from build123d import *

# Parameters (mm, degrees)
SKETCH1_R           = 1.5
BOSS_EXTRUDE1_DEPTH = 3


with BuildPart() as part:
    # Sketch1 → Boss-Extrude1 (new body)
    with BuildSketch(Plane.XY):
        with BuildLine():
            Line((-105, 15), (105, 15))
            ThreePointArc((105, 15), (112.071067812, 12.071067812), (115, 5))
            Line((115, 5), (115, -5))
            ThreePointArc((115, -5), (112.071067812, -12.071067812), (105, -15))
            Line((105, -15), (-105, -15))
            ThreePointArc((-105, -15), (-112.071067812, -12.071067812), (-115, -5))
            Line((-115, -5), (-115, 5))
            ThreePointArc((-115, 5), (-112.071067812, 12.071067812), (-105, 15))
        make_face()
        with Locations((-105, 5)):
            Circle(SKETCH1_R, mode=Mode.SUBTRACT)
        with Locations((-95, 5)):
            Circle(SKETCH1_R, mode=Mode.SUBTRACT)
        with Locations((-85, 5)):
            Circle(SKETCH1_R, mode=Mode.SUBTRACT)
        with Locations((-75, 5)):
            Circle(SKETCH1_R, mode=Mode.SUBTRACT)
        with Locations((-65, 5)):
            Circle(SKETCH1_R, mode=Mode.SUBTRACT)
        with Locations((-55, 5)):
            Circle(SKETCH1_R, mode=Mode.SUBTRACT)
        with Locations((-45, 5)):
            Circle(SKETCH1_R, mode=Mode.SUBTRACT)
        with Locations((-35, 5)):
            Circle(SKETCH1_R, mode=Mode.SUBTRACT)
        with Locations((-25, 5)):
            Circle(SKETCH1_R, mode=Mode.SUBTRACT)
        with Locations((-15, 5)):
            Circle(SKETCH1_R, mode=Mode.SUBTRACT)
        with Locations((-5, 5)):
            Circle(SKETCH1_R, mode=Mode.SUBTRACT)
        with Locations((15, 5)):
            Circle(SKETCH1_R, mode=Mode.SUBTRACT)
        with Locations((25, 5)):
            Circle(SKETCH1_R, mode=Mode.SUBTRACT)
        with Locations((5, 5)):
            Circle(SKETCH1_R, mode=Mode.SUBTRACT)
        with Locations((35, 5)):
            Circle(SKETCH1_R, mode=Mode.SUBTRACT)
        with Locations((45, 5)):
            Circle(SKETCH1_R, mode=Mode.SUBTRACT)
        with Locations((55, 5)):
            Circle(SKETCH1_R, mode=Mode.SUBTRACT)
        with Locations((65, 5)):
            Circle(SKETCH1_R, mode=Mode.SUBTRACT)
        with Locations((75, 5)):
            Circle(SKETCH1_R, mode=Mode.SUBTRACT)
        with Locations((85, 5)):
            Circle(SKETCH1_R, mode=Mode.SUBTRACT)
        with Locations((95, 5)):
            Circle(SKETCH1_R, mode=Mode.SUBTRACT)
        with Locations((-85, -5)):
            Circle(SKETCH1_R, mode=Mode.SUBTRACT)
        with Locations((-75, -5)):
            Circle(SKETCH1_R, mode=Mode.SUBTRACT)
        with Locations((-65, -5)):
            Circle(SKETCH1_R, mode=Mode.SUBTRACT)
        with Locations((-55, -5)):
            Circle(SKETCH1_R, mode=Mode.SUBTRACT)
        with Locations((-45, -5)):
            Circle(SKETCH1_R, mode=Mode.SUBTRACT)
        with Locations((-35, -5)):
            Circle(SKETCH1_R, mode=Mode.SUBTRACT)
        with Locations((-25, -5)):
            Circle(SKETCH1_R, mode=Mode.SUBTRACT)
        with Locations((-15, -5)):
            Circle(SKETCH1_R, mode=Mode.SUBTRACT)
        with Locations((-5, -5)):
            Circle(SKETCH1_R, mode=Mode.SUBTRACT)
        with Locations((5, -5)):
            Circle(SKETCH1_R, mode=Mode.SUBTRACT)
        with Locations((15, -5)):
            Circle(SKETCH1_R, mode=Mode.SUBTRACT)
        with Locations((35, -5)):
            Circle(SKETCH1_R, mode=Mode.SUBTRACT)
        with Locations((45, -5)):
            Circle(SKETCH1_R, mode=Mode.SUBTRACT)
        with Locations((25, -5)):
            Circle(SKETCH1_R, mode=Mode.SUBTRACT)
        with Locations((55, -5)):
            Circle(SKETCH1_R, mode=Mode.SUBTRACT)
        with Locations((65, -5)):
            Circle(SKETCH1_R, mode=Mode.SUBTRACT)
        with Locations((75, -5)):
            Circle(SKETCH1_R, mode=Mode.SUBTRACT)
        with Locations((85, -5)):
            Circle(SKETCH1_R, mode=Mode.SUBTRACT)
        with Locations((95, -5)):
            Circle(SKETCH1_R, mode=Mode.SUBTRACT)
        with Locations((105, -5)):
            Circle(SKETCH1_R, mode=Mode.SUBTRACT)
        with Locations((105, 5)):
            Circle(SKETCH1_R, mode=Mode.SUBTRACT)
        with Locations((-105, -5)):
            Circle(SKETCH1_R, mode=Mode.SUBTRACT)
        with Locations((-95, -5)):
            Circle(SKETCH1_R, mode=Mode.SUBTRACT)
    extrude(amount=BOSS_EXTRUDE1_DEPTH)


solid = part.part
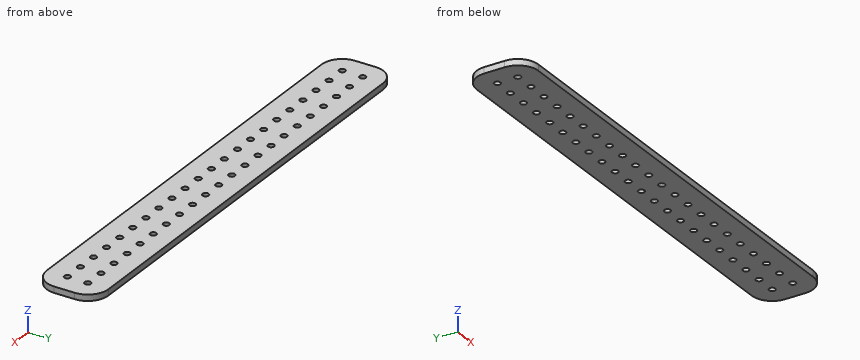
The model under review builds one solid part; all positions refer to its coordinate system, in mm. Round coordinates to 2 decimals unless told otherwise and drop trailing zeros. Use CSV: the item, a comma, the result in double quotes.
(1) Clearance check with a flat-ended pin moving along its axis: P1, Ø3.5, axis at x = 85, y = -5, coming from the -Z side. State where the tip first meets the part, or that it passes through.
Working result:
P1,"stops at z = 0"
(2) For line 1 (Y direction, x = -105, z = 1.95); line 2 (Y direction, x = -35.5, z = 2.3); line 3 (X direction, y = -10.5, z = 1.2), list the stretches that pass through material, from the lowest coordinate up.
Working result:
line 1,"y = -15 to -6.5, -3.5 to 3.5, 6.5 to 15"
line 2,"y = -15 to -6.41, -3.59 to 3.59, 6.41 to 15"
line 3,"x = -113.35 to 113.35"
(3) Take a section at A-A, the plane z = 1.3. State how many separate pieces and enclosed holes the cut face has, plus the area to 3 significant figures.
Working result:
separate pieces,"1"
enclosed holes,"44"
area,"6,500 mm^2"
